Source: CAD feature listing. Evaluate the final solid. Frame: model axes, mm. Face numbers are marked on the shaded views. Coordinates: 2 decimals unless noted, no trailing zeros. Order: outer loops, then holes, each group sorted by start corner. A loop starts at its lowest first (then second) coordinate and runs counter-clockwise, first axis right, second up.
```python
from build123d import *

# Parameters (mm, degrees)
SKETCH_14_R     = 1
EXTRUDE_1_DEPTH = 2


with BuildPart() as part:
    # 草圖14 → 填料-伸長1 (new body)
    with BuildSketch(Plane.XY):
        with BuildLine():
            Line((-33.721403204, -5), (-33.721403204, -7))
            ThreePointArc((-33.721403204, -7), (-34.014296423, -7.707106781), (-34.721403204, -8))
            Line((-34.721403204, -8), (-36.721403204, -8))
            Line((-36.721403204, -8), (-36.721403204, -16))
            Line((-36.721403204, -16), (-34.721403204, -16))
            ThreePointArc((-34.721403204, -16), (-34.014296423, -16.292893219), (-33.721403204, -17))
            Line((-33.721403204, -17), (-33.721403204, -19))
            ThreePointArc((-33.721403204, -19), (-34.014296423, -19.707106781), (-34.721403204, -20))
            Line((-34.721403204, -20), (-36.721403204, -20))
            Line((-36.721403204, -20), (-36.721403204, -24))
            Line((-36.721403204, -24), (14.878596796, -24))
            Line((14.878596796, -24), (14.878596796, -20))
            Line((14.878596796, -20), (12.878596796, -20))
            ThreePointArc((12.878596796, -20), (12.171490014, -19.707106781), (11.878596796, -19))
            Line((11.878596796, -19), (11.878596796, -17))
            ThreePointArc((11.878596796, -17), (12.171490014, -16.292893219), (12.878596796, -16))
            Line((12.878596796, -16), (14.878596796, -16))
            Line((14.878596796, -16), (14.878596796, -8))
            Line((14.878596796, -8), (12.878596796, -8))
            ThreePointArc((12.878596796, -8), (12.171490014, -7.707106781), (11.878596796, -7))
            Line((11.878596796, -7), (11.878596796, -5))
            ThreePointArc((11.878596796, -5), (12.171490014, -4.292893219), (12.878596796, -4))
            Line((12.878596796, -4), (14.878596796, -4))
            Line((14.878596796, -4), (14.878596796, 0))
            Line((14.878596796, 0), (-36.721403204, 0))
            Line((-36.721403204, 0), (-36.721403204, -4))
            Line((-36.721403204, -4), (-34.721403204, -4))
            ThreePointArc((-34.721403204, -4), (-34.014296423, -4.292893219), (-33.721403204, -5))
        make_face()
        with Locations((10.878596796, -14)):
            Circle(SKETCH_14_R, mode=Mode.SUBTRACT)
        with Locations((5.378124186, -14)):
            Circle(SKETCH_14_R, mode=Mode.SUBTRACT)
        with Locations((5.378124186, -22)):
            Circle(SKETCH_14_R, mode=Mode.SUBTRACT)
        with Locations((10.878596796, -22)):
            Circle(SKETCH_14_R, mode=Mode.SUBTRACT)
        with Locations((-26.621875814, -14)):
            Circle(SKETCH_14_R, mode=Mode.SUBTRACT)
        with Locations((-32.721875814, -14)):
            Circle(SKETCH_14_R, mode=Mode.SUBTRACT)
        with Locations((-32.721875814, -22)):
            Circle(SKETCH_14_R, mode=Mode.SUBTRACT)
        with Locations((-26.621875814, -22)):
            Circle(SKETCH_14_R, mode=Mode.SUBTRACT)
        with Locations((5.378124186, -2)):
            Circle(SKETCH_14_R, mode=Mode.SUBTRACT)
        with Locations((5.378124186, -10)):
            Circle(SKETCH_14_R, mode=Mode.SUBTRACT)
        with Locations((10.878596796, -10)):
            Circle(SKETCH_14_R, mode=Mode.SUBTRACT)
        with Locations((-32.721403204, -2)):
            Circle(SKETCH_14_R, mode=Mode.SUBTRACT)
        with Locations((-26.621875814, -2)):
            Circle(SKETCH_14_R, mode=Mode.SUBTRACT)
        with Locations((-32.721403204, -10)):
            Circle(SKETCH_14_R, mode=Mode.SUBTRACT)
        with Locations((-26.621875814, -10)):
            Circle(SKETCH_14_R, mode=Mode.SUBTRACT)
        with Locations((10.878596796, -2)):
            Circle(SKETCH_14_R, mode=Mode.SUBTRACT)
        with BuildLine():
            Line((-30.621875814, -4), (-28.621875814, -4))
            ThreePointArc((-28.621875814, -4), (-27.914769033, -4.292893219), (-27.621875814, -5))
            Line((-27.621875814, -5), (-27.621875814, -7))
            ThreePointArc((-27.621875814, -7), (-27.914769033, -7.707106781), (-28.621875814, -8))
            Line((-28.621875814, -8), (-30.621875814, -8))
            ThreePointArc((-30.621875814, -8), (-31.328982596, -7.707106781), (-31.621875814, -7))
            Line((-31.621875814, -7), (-31.621875814, -5))
            ThreePointArc((-31.621875814, -5), (-31.328982596, -4.292893219), (-30.621875814, -4))
        make_face(mode=Mode.SUBTRACT)
        with BuildLine():
            Line((-27.621875814, -17), (-27.621875814, -19))
            ThreePointArc((-27.621875814, -19), (-27.914769033, -19.707106781), (-28.621875814, -20))
            Line((-28.621875814, -20), (-30.621875814, -20))
            ThreePointArc((-30.621875814, -20), (-31.328982596, -19.707106781), (-31.621875814, -19))
            Line((-31.621875814, -19), (-31.621875814, -17))
            ThreePointArc((-31.621875814, -17), (-31.328982596, -16.292893219), (-30.621875814, -16))
            Line((-30.621875814, -16), (-28.621875814, -16))
            ThreePointArc((-28.621875814, -16), (-27.914769033, -16.292893219), (-27.621875814, -17))
        make_face(mode=Mode.SUBTRACT)
    extrude(amount=EXTRUDE_1_DEPTH)


solid = part.part
```
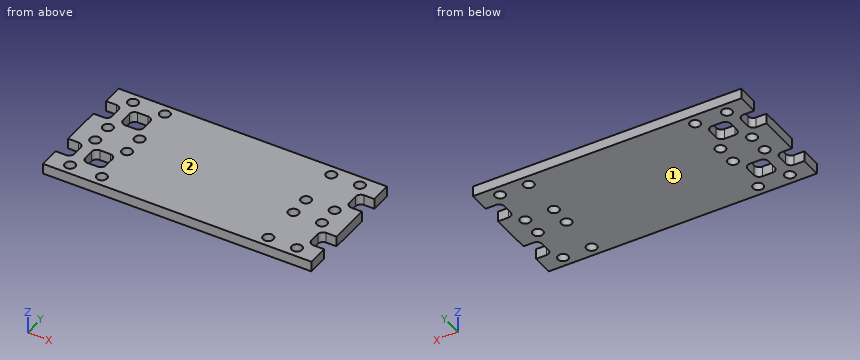
1. Section query A-A on y = -2. Return loops of the section in (x, z), plus the area to 3 significant figures.
Findings:
outline: (-36.72, 0) - (-33.72, 0) - (-33.72, 2) - (-36.72, 2) - close; (-31.72, 0) - (-27.62, 0) - (-27.62, 2) - (-31.72, 2) - close; (-25.62, 0) - (4.38, 0) - (4.38, 2) - (-25.62, 2) - close; (6.38, 0) - (9.88, 0) - (9.88, 2) - (6.38, 2) - close; (11.88, 0) - (14.88, 0) - (14.88, 2) - (11.88, 2) - close
area: 87.2 mm2
2. Ray query, line 1 (Y direction, x = -30.5, z = 0.3); line 2 (Y direction, x = -27, z = 0.75); line 3 (Y direction, x = -26, z = 1.8). Return the intervals inside material, ascending.
Findings:
line 1: y = -24 to -20, -16 to -8, -4 to 0
line 2: y = -24 to -22.93, -21.07 to -14.93, -13.07 to -10.93, -9.07 to -2.93, -1.07 to 0
line 3: y = -24 to -22.78, -21.22 to -14.78, -13.22 to -10.78, -9.22 to -2.78, -1.22 to 0
3. Section query B-B on z = 0.5. Count the separate pieces of the cut face and the enclosed holes in it, plus the area to 3 significant figures.
Findings:
separate pieces: 1
enclosed holes: 18
area: 1,110 mm2
4. Draft query along Z for the marked faces 1 and 2. Return one class per face: released by +Z, released by -Z, zero draft, split by the parting line, or undercut.
Findings:
face 1: released by -Z
face 2: released by +Z
